from build123d import *

# Parameters (mm, degrees)
BASPROSKE_W        = 5
BASPROSKE_H        = 15.75
TOOTHCUT_DEPTH     = 23.828162432
TEETHCUTS_COUNT    = 19
TEETHCUTS_ANGLE    = 341.052631579
BORSKE_R           = 0.4
BORE_DEPTH         = 50.0000508
CUT_EXTRUDE1_DEPTH = 23.81496003


with BuildPart() as part:
    # BasProSke → Base-Revolve (revolve)
    with BuildSketch(Plane(origin=(0, 0, 0), x_dir=(1, 0, 0), z_dir=(0, 1, 0)), mode=Mode.PRIVATE) as base_revolve_sk:
        with Locations((2.5, 7.875)):
            Rectangle(BASPROSKE_W, BASPROSKE_H)
    revolve(base_revolve_sk.sketch.rotate(Axis((-10, 0, 0), (1, 0, 0)), 180), axis=Axis((-10, 0, 0), (1, 0, 0)))

    # TooCutSke → ToothCut (cut, through all)
    with BuildSketch(Plane(origin=(0, 0, 0), x_dir=(0, 0, -1), z_dir=(1, 0, 0))):
        with BuildLine():
            ThreePointArc((0.885187307, 12.34229798), (0, 12.374), (-0.885187307, 12.34229798))
            ThreePointArc((-0.885187307, 12.34229798), (-1.228281365, 14.084307739), (-2.090723145, 15.636243855))
            ThreePointArc((-2.090723145, 15.636243855), (0, 15.7754), (2.090723145, 15.636243855))
            ThreePointArc((2.090723145, 15.636243855), (1.228281365, 14.084307739), (0.885187307, 12.34229798))
        make_face()
    toothcut = extrude(amount=TOOTHCUT_DEPTH, mode=Mode.SUBTRACT)

    # TeethCuts: ToothCut ×19 about axis
    teethcuts_axis = Axis((-10, 0, 0), (1, 0, 0))
    for i in range(1, TEETHCUTS_COUNT):
        add(toothcut.rotate(teethcuts_axis, i * TEETHCUTS_ANGLE / (TEETHCUTS_COUNT - 1)), mode=Mode.SUBTRACT)

    # BorSke → Bore (cut, symmetric)
    with BuildSketch(Plane(origin=(0, 0, 0), x_dir=(0, 0, -1), z_dir=(1, 0, 0))):
        with Locations(Location((0, 0, 0), (0, 0, 180))):
            Circle(BORSKE_R)
    extrude(amount=BORE_DEPTH, both=True, mode=Mode.SUBTRACT)

    # Sketch1 → Cut-Extrude1 (cut, through all)
    with BuildSketch(Plane(origin=(5, 0, 0), x_dir=(0, 0, -1), z_dir=(1, 0, 0))):
        with BuildLine():
            Line((1.560589416, 1.250823998), (-1.560589416, 1.250823998))
            ThreePointArc((-1.560589416, 1.250823998), (-0.66288052, -1.886952415), (2, 0))
            ThreePointArc((2, 0), (1.886952415, 0.66288052), (1.560589416, 1.250823998))
        make_face()
    extrude(amount=-CUT_EXTRUDE1_DEPTH, mode=Mode.SUBTRACT)


solid = part.part
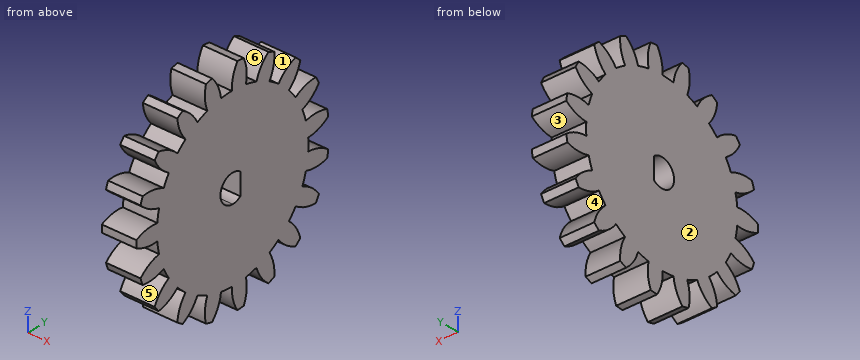
The listing builds one solid part. Answer for the finished solid, in the listing's coordinates (mm). Face numbers are marked on the shaded views. A direction names the side the tool comes from. Give positions to 0.01 mm unless a question says otherwise; leave off trailing zeros. Order: outer loops, then holes, each group sorted by start corner. A loop starts at its lowest first (then second) coordinate and runs counter-clockwise, first axis right, second up. Notation, with made-up numbers: (63.25, -30.75) -> (101.25, -30.75) arc R16 cw to (101.25, -9.75) -> close; hole circle Ø3 at (20.25, 66). An arc over 180 degrees is marked (long way). Put each result on its own line as item: value.
Item 1: For a pull along Y with two mould halves and no side action, classify the marked faces 1, 2 and 3 as released by +Y, released by -Y, zero draft, split by the parting line, or undercut.
Established:
face 1: undercut
face 2: zero draft
face 3: released by +Y
Item 2: For the marked faces 4, 5 and 6, determine the directions among +Z, -Z, +X, -X, +Y, -Y from which every point of the face is accessible in a straight line to the end or side of a thin tool.
Established:
face 4: +X, -X
face 5: +X, -X, -Y
face 6: +Z, +X, -X
Item 3: A cutting plane is placed at C-C on y = 5. Give the vertices of the cut face in (x, z), plus the area to 3 significant figures.
Established:
outline: (0, -13.81) -> (5, -13.81) -> (5, 13.81) -> (0, 13.81) -> close
area: 138 mm^2
Item 4: A cutting plane is placed at B-B on z = 7.5. Give the vertices of the cut face in (x, y).
Established:
outline: (0, -11.53) -> (5, -11.53) -> (5, 9.84) -> (0, 9.84) -> close; (0, 11.38) -> (5, 11.38) -> (5, 13.85) -> (0, 13.85) -> close
Item 5: Given P1, Ø1.5, axis at x = 1.5, y = -6, coming from the -Z side; P2, Ø2, axis at x = 4, y = -7.5, coming from the +Z side, each flat-ended and moving along its own axis, determine where each tip first touches the part or whether it passes through.
Established:
P1: stops at z = -12.37
P2: stops at z = 13.47
Item 6: A cutting plane is placed at D-D on z = -4. Give the vertices of the cut face in (x, y).
Established:
outline: (0, -14.39) -> (5, -14.39) -> (5, 11.71) -> (0, 11.71) -> close
Item 7: Straight lines are drawn through the part: line 1 (Z direction, x = 0.65, y = 10.5); line 2 (Y direction, x = 3, z = 0); line 3 (Y direction, x = 4.1, z = -13). For each, find the intervals that lie inside material, in ascending order.
Established:
line 1: z = -11.74 to -9.86, -7.03 to 7.03, 9.86 to 11.74
line 2: y = -15.75 to -2, 1.25 to 12.37
line 3: y = -8.89 to -7.45, -4.49 to -2.05, -0.13 to 2.28, 4.43 to 6.77
Item 8: A cutting plane is placed at A-A on z = 0. Give the vertices of the cut face in (x, y).
Established:
outline: (0, -15.75) -> (5, -15.75) -> (5, -2) -> (0, -2) -> close; (0, 1.25) -> (5, 1.25) -> (5, 12.37) -> (0, 12.37) -> close
